Autodesk Inventor part; units mm, degrees
ref_plane "YZ Plane" through (0, 0, 0) normal (1, 0, 0) x (0, 1, 0)
ref_plane "XZ Plane" through (0, 0, 0) normal (0, 1, 0) x (-1, 0, 0)
ref_plane "XY Plane" through (0, 0, 0) normal (0, 0, 1) x (1, 0, 0)
sketch "Sketch1" plane through (0, 0, 0) normal (0, 0, 1) x (1, 0, 0)
  line L0 (-20, 0) -> (20, 0)
  line L1 (20, 0) -> (20, 10)
  line L2 (20, 10) -> (-20, 10)
  line L3 (-20, 10) -> (-20, 0)
  point P0 (0, 0)
  point P1 (0, 0)
  dimension "d0" = 40
  dimension "d1" = 10
extrude "Extrusion1" add sketch "Sketch1" against normal blind 30
fillet "Fillet1" radius 4 2 edges at (20, 10, -15) (-20, 10, -15)
sketch "Sketch2" plane through (0, 0, 0) normal (0, 0, 1) x (1, 0, 0)
  arc A0 (-16, 10) -> (-20, 6) centre (-16, 6) ccw
  line L0 (-20, 6) -> (-20, 0)
  line L1 (-20, 0) -> (20, 0)
  line L2 (20, 0) -> (20, 6)
  arc A1 (20, 6) -> (16, 10) centre (16, 6) ccw
  line L3 (16, 10) -> (-16, 10)
  line L4 (-20, 0) -> (20, 0)
  point P0 (0, 0)
  point P1 (-14, 6)
  point P2 (14, 6)
  point P3 (0, 0)
  dimension "d12" = 28
  dimension "d13" = 14
hole "Hole1" at (-14, 6, 0) at (14, 6, 0) direction (0, 0, -1) diameter 4.134 depth 30
properties part number "02A" material "Aluminum 6061"
Geometry: final body of the model. Coordinates: model frame, mm. Round coordinates to 2 decimals unless told otherwise and drop trailing zeros. Loops run counter-clockwise (first coordinate to the right, second up) from the corner with the lowest first, then second, coordinate; pieces in that order, holes last. Notation, with made-up numbers: (34.25, 89.5) - (54.25, 89.5) arc R12 cw to (54.25, 97.5) - close; hole circle Ø9 at (84, 37). An arc over 180 degrees is marked (long way). Write each question's results on one line, items separated by ' | '. Start each with the question number.
1) Cut plane A-A on x = -14. Return loops of the section in (y, z), then the cut area to 3 significant figures.
2) Cut plane B-B on y = 5.25. Return loops of the section in (x, z), then the cut area to 3 significant figures.
3) First-contact query: P1, Ø5, axis at x = 14, y = 6, coming from the +Z side; P2, Ø1, axis at y = 7, z = -3, coming from the +X side. Flat tips, straight axial feed; report the tip coordinate or a pass-through.
4) Line query: probe 1 along X at (y, z) = (6, -17.25); probe 2 along X at (y, z) = (6.5, -22.25); probe 3 along Y at (x, z) = (14, -22.75). Output: solid intervals per line, ascending. Write a range as [from, to].
5) Cut plane C-C on z = -8.5. Return loops of the section in (x, y).
Verdict:
1) outline: (0, -30) - (3.93, -30) - (3.93, 0) - (0, 0) - close; (8.07, -30) - (10, -30) - (10, 0) - (8.07, 0) - close | area: 176 mm2
2) outline: (-20, -30) - (-15.93, -30) - (-15.93, 0) - (-20, 0) - close; (-12.07, -30) - (12.07, -30) - (12.07, 0) - (-12.07, 0) - close; (15.93, -30) - (20, -30) - (20, 0) - (15.93, 0) - close | area: 969 mm2
3) P1: stops at z = 0 | P2: stops at x = 19.97
4) probe 1: x = [-20, -16.07], [-11.93, 11.93], [16.07, 20] | probe 2: x = [-19.97, -16.01], [-11.99, 11.99], [16.01, 19.97] | probe 3: y = [0, 3.93], [8.07, 10]
5) outline: (-20, 0) - (20, 0) - (20, 6) arc R4 ccw to (16, 10) - (-16, 10) arc R4 ccw to (-20, 6) - close; hole circle Ø4.13 at (-14, 6); hole circle Ø4.13 at (14, 6)
